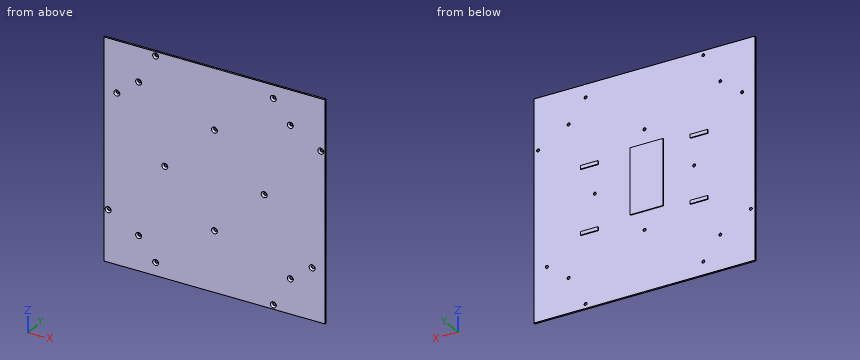
from build123d import *

# Parameters (mm, degrees)
SKETCH1_W                                      = 254
SKETCH1_H                                      = 254
BOSS_EXTRUDE1_DEPTH                            = 1.016
CSK_FOR_M3_FLAT_HEAD_MACHINE_SCREW2_AT_2_COUNT = 2
CSK_FOR_M3_FLAT_HEAD_MACHINE_SCREW2_AT_2_PITCH = 70.359789653
CSK_FOR_M3_FLAT_HEAD_MACHINE_SCREW2_AT_3_COUNT = 2
CSK_FOR_M3_FLAT_HEAD_MACHINE_SCREW2_AT_3_PITCH = 184.933771929
CSK_FOR_M3_FLAT_HEAD_MACHINE_SCREW2_AT_4_COUNT = 2
CSK_FOR_M3_FLAT_HEAD_MACHINE_SCREW2_AT_4_PITCH = 234
CSK_FOR_M3_FLAT_HEAD_MACHINE_SCREW2_AT_5_COUNT = 2
CSK_FOR_M3_FLAT_HEAD_MACHINE_SCREW2_AT_5_PITCH = 261.535848403
CSK_FOR_M3_FLAT_HEAD_MACHINE_SCREW2_AT_6_COUNT = 2
CSK_FOR_M3_FLAT_HEAD_MACHINE_SCREW2_AT_6_PITCH = 184.933771929
CSK_FOR_M3_FLAT_HEAD_MACHINE_SCREW2_AT_7_COUNT = 2
CSK_FOR_M3_FLAT_HEAD_MACHINE_SCREW2_AT_7_PITCH = 135.369863707
CSK_FOR_M3_FLAT_HEAD_MACHINE_SCREW2_AT_8_COUNT = 2
CSK_FOR_M3_FLAT_HEAD_MACHINE_SCREW2_AT_8_PITCH = 261.018198599
SKETCH10_W                                     = 20
SKETCH10_H                                     = 4
SKETCH10_W_2                                   = 38
SKETCH10_H_2                                   = 76
BOSS_EXTRUDE2_DEPTH                            = 1
CSK_FOR_M3_FLAT_HEAD_MACHINE_SCREW3_AT_2_COUNT = 2
CSK_FOR_M3_FLAT_HEAD_MACHINE_SCREW3_AT_2_PITCH = 80.610173055
CSK_FOR_M3_FLAT_HEAD_MACHINE_SCREW3_AT_3_COUNT = 2
CSK_FOR_M3_FLAT_HEAD_MACHINE_SCREW3_AT_3_PITCH = 80.610173055
CSK_FOR_M3_FLAT_HEAD_MACHINE_SCREW3_AT_4_COUNT = 2
CSK_FOR_M3_FLAT_HEAD_MACHINE_SCREW3_AT_4_PITCH = 114
CSK_FOR_M3_FLAT_HEAD_MACHINE_SCREW3_AT_5_COUNT = 2
CSK_FOR_M3_FLAT_HEAD_MACHINE_SCREW3_AT_5_PITCH = 168.240898714
CSK_FOR_M3_FLAT_HEAD_MACHINE_SCREW3_AT_6_COUNT = 2
CSK_FOR_M3_FLAT_HEAD_MACHINE_SCREW3_AT_6_PITCH = 92.027169901
CSK_FOR_M3_FLAT_HEAD_MACHINE_SCREW3_AT_7_COUNT = 2
CSK_FOR_M3_FLAT_HEAD_MACHINE_SCREW3_AT_7_PITCH = 92.027169901
CSK_FOR_M3_FLAT_HEAD_MACHINE_SCREW3_AT_8_COUNT = 2
CSK_FOR_M3_FLAT_HEAD_MACHINE_SCREW3_AT_8_PITCH = 168.240898714


with BuildPart() as part:
    # Sketch1 → Boss-Extrude1 (new, symmetric)
    with BuildSketch(Plane(origin=(0, 0, 0), x_dir=(1, 0, 0), z_dir=(0, 1, 0))):
        Rectangle(SKETCH1_W, SKETCH1_H)
    extrude(amount=BOSS_EXTRUDE1_DEPTH, both=True)

    # Sketch9 → CSK for M3 Flat Head Machine Screw2 (revolve, cut)
    with BuildSketch(Plane(origin=(-67.5, -1.016, -112), x_dir=(0, 0, -1), z_dir=(1, 0, 0))):
        Polygon((0, 0), (0, 2.032), (1.7, 2.032), (1.7, 1.7), (3.4, 0), align=None)
    csk_for_m3_flat_head_machine_screw2 = revolve(axis=Axis((-67.5, -7.366, -112), (0, 1, 0)), mode=Mode.SUBTRACT)

    # CSK for M3 Flat Head Machine Screw2 at 2: CSK for M3 Flat Head Machine Screw2 ×2
    with Locations(*[Vector(-0.7745901496986006, 0, 0.6324635167263798) * (i * CSK_FOR_M3_FLAT_HEAD_MACHINE_SCREW2_AT_2_PITCH) for i in range(1, CSK_FOR_M3_FLAT_HEAD_MACHINE_SCREW2_AT_2_COUNT)]):
        add(csk_for_m3_flat_head_machine_screw2, mode=Mode.SUBTRACT)

    # CSK for M3 Flat Head Machine Screw2 at 3: CSK for M3 Flat Head Machine Screw2 ×2
    with Locations(*[Vector(-0.24062668238341703, 0, 0.9706177412994006) * (i * CSK_FOR_M3_FLAT_HEAD_MACHINE_SCREW2_AT_3_PITCH) for i in range(1, CSK_FOR_M3_FLAT_HEAD_MACHINE_SCREW2_AT_3_COUNT)]):
        add(csk_for_m3_flat_head_machine_screw2, mode=Mode.SUBTRACT)

    # CSK for M3 Flat Head Machine Screw2 at 4: CSK for M3 Flat Head Machine Screw2 ×2
    with Locations(*[(0, 0, i * CSK_FOR_M3_FLAT_HEAD_MACHINE_SCREW2_AT_4_PITCH) for i in range(1, CSK_FOR_M3_FLAT_HEAD_MACHINE_SCREW2_AT_4_COUNT)]):
        add(csk_for_m3_flat_head_machine_screw2, mode=Mode.SUBTRACT)

    # CSK for M3 Flat Head Machine Screw2 at 5: CSK for M3 Flat Head Machine Screw2 ×2
    with Locations(*[Vector(0.5161816279650405, 0, 0.856479145660512) * (i * CSK_FOR_M3_FLAT_HEAD_MACHINE_SCREW2_AT_5_PITCH) for i in range(1, CSK_FOR_M3_FLAT_HEAD_MACHINE_SCREW2_AT_5_COUNT)]):
        add(csk_for_m3_flat_head_machine_screw2, mode=Mode.SUBTRACT)

    # CSK for M3 Flat Head Machine Screw2 at 6: CSK for M3 Flat Head Machine Screw2 ×2
    with Locations(*[Vector(0.9706177412994007, 0, 0.2406266823834169) * (i * CSK_FOR_M3_FLAT_HEAD_MACHINE_SCREW2_AT_6_PITCH) for i in range(1, CSK_FOR_M3_FLAT_HEAD_MACHINE_SCREW2_AT_6_COUNT)]):
        add(csk_for_m3_flat_head_machine_screw2, mode=Mode.SUBTRACT)

    # CSK for M3 Flat Head Machine Screw2 at 7: CSK for M3 Flat Head Machine Screw2 ×2
    with Locations(*[Vector(0.997267754456709, 0, -0.07387168551531198) * (i * CSK_FOR_M3_FLAT_HEAD_MACHINE_SCREW2_AT_7_PITCH) for i in range(1, CSK_FOR_M3_FLAT_HEAD_MACHINE_SCREW2_AT_7_COUNT)]):
        add(csk_for_m3_flat_head_machine_screw2, mode=Mode.SUBTRACT)

    # CSK for M3 Flat Head Machine Screw2 at 8: CSK for M3 Flat Head Machine Screw2 ×2
    with Locations(*[Vector(0.7260030182452614, 0, 0.687691513324667) * (i * CSK_FOR_M3_FLAT_HEAD_MACHINE_SCREW2_AT_8_PITCH) for i in range(1, CSK_FOR_M3_FLAT_HEAD_MACHINE_SCREW2_AT_8_COUNT)]):
        add(csk_for_m3_flat_head_machine_screw2, mode=Mode.SUBTRACT)

    # Sketch10 → Boss-Extrude2 (add)
    with BuildSketch(Plane(origin=(0, 1.016, 0), x_dir=(1, 0, 0), z_dir=(0, 1, 0))):
        with Locations((-62.95, 40.95)):
            Rectangle(SKETCH10_W, SKETCH10_H)
        with Locations((62.95, 40.95)):
            Rectangle(SKETCH10_W, SKETCH10_H)
        with Locations((-62.95, -33.95)):
            Rectangle(SKETCH10_W, SKETCH10_H)
        with Locations((62.95, -33.95)):
            Rectangle(SKETCH10_W, SKETCH10_H)
        with Locations((-2.95, -2.05)):
            Rectangle(SKETCH10_W_2, SKETCH10_H_2)
    extrude(amount=BOSS_EXTRUDE2_DEPTH)

    # Sketch13 → CSK for M3 Flat Head Machine Screw3 (revolve, cut)
    with BuildSketch(Plane(origin=(0, -1.016, 57), x_dir=(0, 0, -1), z_dir=(1, 0, 0))):
        Polygon((0, 0), (0, 3.032), (1.7, 3.032), (1.7, 1.7), (3.4, 0), align=None)
    csk_for_m3_flat_head_machine_screw3 = revolve(axis=Axis((0, -7.366, 57), (0, 1, 0)), mode=Mode.SUBTRACT)

    # CSK for M3 Flat Head Machine Screw3 at 2: CSK for M3 Flat Head Machine Screw3 ×2
    with Locations(*[Vector(0.7071067811865476, 0, -0.7071067811865476) * (i * CSK_FOR_M3_FLAT_HEAD_MACHINE_SCREW3_AT_2_PITCH) for i in range(1, CSK_FOR_M3_FLAT_HEAD_MACHINE_SCREW3_AT_2_COUNT)]):
        add(csk_for_m3_flat_head_machine_screw3, mode=Mode.SUBTRACT)

    # CSK for M3 Flat Head Machine Screw3 at 3: CSK for M3 Flat Head Machine Screw3 ×2
    with Locations(*[Vector(-0.7071067811865476, 0, -0.7071067811865476) * (i * CSK_FOR_M3_FLAT_HEAD_MACHINE_SCREW3_AT_3_PITCH) for i in range(1, CSK_FOR_M3_FLAT_HEAD_MACHINE_SCREW3_AT_3_COUNT)]):
        add(csk_for_m3_flat_head_machine_screw3, mode=Mode.SUBTRACT)

    # CSK for M3 Flat Head Machine Screw3 at 4: CSK for M3 Flat Head Machine Screw3 ×2
    with Locations(*[(0, 0, -i * CSK_FOR_M3_FLAT_HEAD_MACHINE_SCREW3_AT_4_PITCH) for i in range(1, CSK_FOR_M3_FLAT_HEAD_MACHINE_SCREW3_AT_4_COUNT)]):
        add(csk_for_m3_flat_head_machine_screw3, mode=Mode.SUBTRACT)

    # CSK for M3 Flat Head Machine Screw3 at 5: CSK for M3 Flat Head Machine Screw3 ×2
    with Locations(*[Vector(-0.5171156399255817, 0, -0.8559155419457904) * (i * CSK_FOR_M3_FLAT_HEAD_MACHINE_SCREW3_AT_5_PITCH) for i in range(1, CSK_FOR_M3_FLAT_HEAD_MACHINE_SCREW3_AT_5_COUNT)]):
        add(csk_for_m3_flat_head_machine_screw3, mode=Mode.SUBTRACT)

    # CSK for M3 Flat Head Machine Screw3 at 6: CSK for M3 Flat Head Machine Screw3 ×2
    with Locations(*[Vector(-0.9453729816262721, 0, 0.32599068331940434) * (i * CSK_FOR_M3_FLAT_HEAD_MACHINE_SCREW3_AT_6_PITCH) for i in range(1, CSK_FOR_M3_FLAT_HEAD_MACHINE_SCREW3_AT_6_COUNT)]):
        add(csk_for_m3_flat_head_machine_screw3, mode=Mode.SUBTRACT)

    # CSK for M3 Flat Head Machine Screw3 at 7: CSK for M3 Flat Head Machine Screw3 ×2
    with Locations(*[Vector(0.9453729816262721, 0, 0.32599068331940434) * (i * CSK_FOR_M3_FLAT_HEAD_MACHINE_SCREW3_AT_7_PITCH) for i in range(1, CSK_FOR_M3_FLAT_HEAD_MACHINE_SCREW3_AT_7_COUNT)]):
        add(csk_for_m3_flat_head_machine_screw3, mode=Mode.SUBTRACT)

    # CSK for M3 Flat Head Machine Screw3 at 8: CSK for M3 Flat Head Machine Screw3 ×2
    with Locations(*[Vector(0.5171156399255817, 0, -0.8559155419457904) * (i * CSK_FOR_M3_FLAT_HEAD_MACHINE_SCREW3_AT_8_PITCH) for i in range(1, CSK_FOR_M3_FLAT_HEAD_MACHINE_SCREW3_AT_8_COUNT)]):
        add(csk_for_m3_flat_head_machine_screw3, mode=Mode.SUBTRACT)


solid = part.part
Work out the finished part from the listing and answer in its coordinate system (mm). Give positions to 0.01 mm unless a question says otherwise; leave off trailing zeros. Order: outer loops, then holes, each group sorted by start corner. A loop starts at its lowest first (then second) coordinate and runs counter-clockwise, first axis right, second up. Notation, with made-up numbers: (35.25, 52) -> (40.25, 52) arc R21 cw to (40.25, 69) -> close; hole circle Ø10 at (29, 20). An arc over 180 degrees is marked (long way). Answer as a JSON object with one key per item and string values. Group by question number.
1. Section B-B on x = -12 is taken. Determine the outline of the cut face in (y, z), plus the area to 3 significant figures.
2. Consider line 1 along Z through (x, y) = (0, 0.8); line 2 along X through (y, z) = (0.8, 67.5); line 3 along X through (y, z) = (0.9, 87). Determine where each line is inside the solid, lowest interval first. Write a range as [from, to].
3. Flat-ended cylindrical pins translate along their axes: pin 1 Ø0.5 at (x, y) = (65, 1.5) entering from -Z; pin 2 Ø3 at (x, z) = (57, 0) entering from -Y; pin 3 Ø4.5 at (x, z) = (-67.5, -112) entering from -Y; pin 4 Ø1.1 at (x, y) = (-63, 1.5) entering from -Z. Find the tip coordinate at first contact, or state that the pin passes through.
4. Section D-D on x = -42 is taken. Determine the outline of the cut face in (y, z).
5. Section C-C on z = 96.5 is taken. Determine the outline of the cut face in (x, y), plus the area to 3 significant figures.
6. Section A-A on z = 19 is taken. Determine the outline of the cut face in (x, y).
Result sheet:
{
 "1": {"outline": "(-1.02, -127) -> (1.02, -127) -> (1.02, -35.95) -> (2.02, -35.95) -> (2.02, 40.05) -> (1.02, 40.05) -> (1.02, 127) -> (-1.02, 127) -> close", "area": "592 mm^2"},
 "2": {"line 1": "z = [-127, -58.7], [-55.3, 55.3], [58.7, 127]", "line 2": "x = [-127, -113.7], [-110.3, 120.3], [123.7, 127]", "line 3": "x = [-127, -88.7], [-85.3, 85.3], [88.7, 127]"},
 "3": {"pin 1": "stops at z = -42.95", "pin 2": "passes through", "pin 3": "stops at y = 0.13", "pin 4": "stops at z = -127"},
 "4": {"outline": "(-1.02, -127) -> (1.02, -127) -> (1.02, 127) -> (-1.02, 127) -> close"},
 "5": {"outline": "(-127, -1.02) -> (127, -1.02) -> (127, 1.02) -> (-127, 1.02) -> close", "area": "516 mm^2"},
 "6": {"outline": "(-127, -1.02) -> (127, -1.02) -> (127, 1.02) -> (16.05, 1.02) -> (16.05, 2.02) -> (-21.95, 2.02) -> (-21.95, 1.02) -> (-127, 1.02) -> close"}
}
